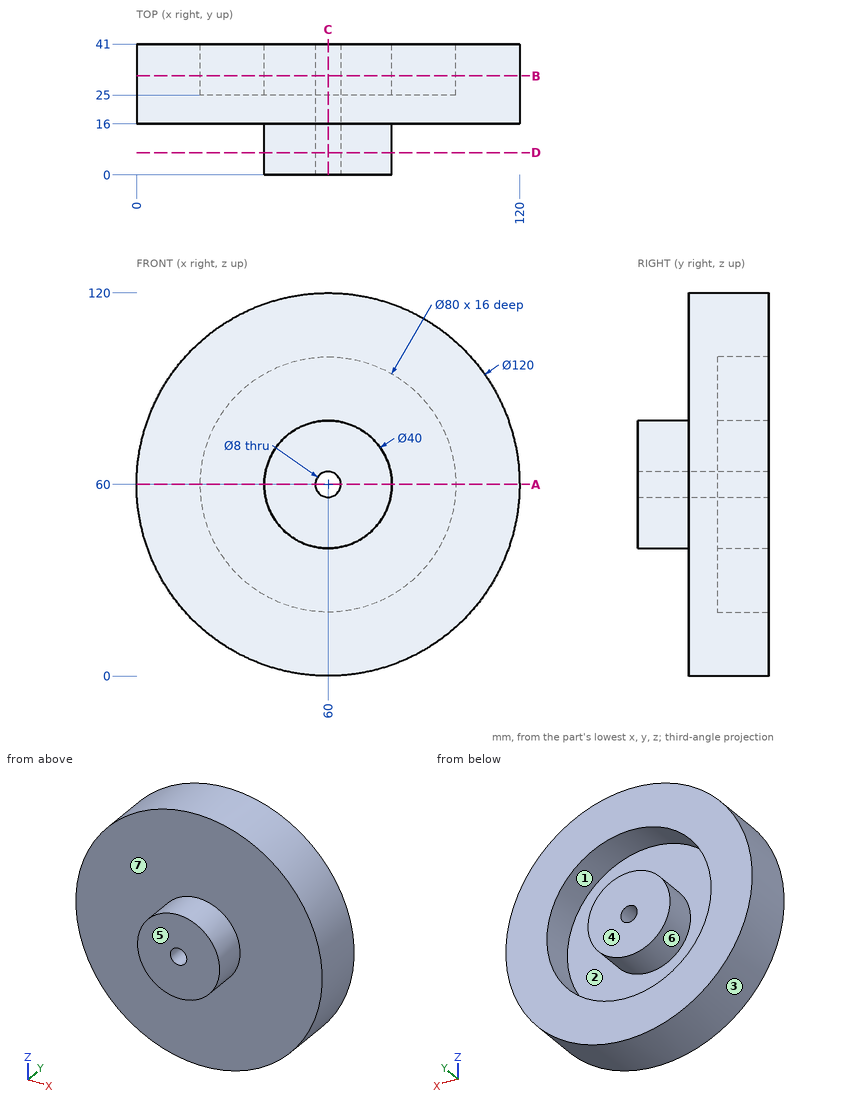
The drawing under review shows one solid part. Ordinate dimensions are in mm from its lowest x, y, z. A direction names the side the tool comes from. Round coordinates to 2 decimals unless told otherwise and drop trailing zeros. Write each loop counter-clockwise with the first axis right and the second up, starting at its lowest first coordinate (ties: lowest second). Pieces come first, ordered by that corner, then holes.
(1) We need section A-A on z = 60. Give the boundary of the cut face in (x, y).
(2) Machinability: for the marked faces 5, 6 and 7, which of the approach directions +Z, -Z, +X, -X, +Y, -Y give a long, thin tool a straight path to every point of the face, cutting with its end or side? Answer none if there is none.
(3) Wall thickness on L1, parallel to X at y = 30.5, z = 60; L2, parallel to X at y = 12, z = 60; L3, parallel to Y at x = 8.5, z = 67.5: over which ranges is each line inside the solid? List them lowest first.
(4) Mouldability with a two-part tool opening along X and no side actions: class the marked faces 1, 2, 3 and 4 as +X half, -X half, draft (parallel to the pull), parting line (faces both ways), or undercut.
(5) We need section D-D on y = 7. Give the boundary of the cut face in (x, z), and give its area (3 significant figures).
(6) Insertion check: pin 1 (1.5 mm diameter, centred on x = 100, y = 22, fed in from -Z); pin 2 (12 mm diameter, centred on x = 12, z = 73, fed in from -Y); pin 3 (6 mm diameter, centred on x = 50.5, y = 9, fed in from -Z). Each pin has a flat end and moves straight along its axis. Give the tip position at first contact, or say it passes through.
(7) We need section C-C on x = 60. Give the boundary of the cut face in (y, z).
(8) We need section B-B on y = 31. Give the boundary of the cut face in (x, z), and give its area (3 significant figures).
Findings below:
1. outline: (0, 16) - (40, 16) - (40, 0) - (56, 0) - (56, 41) - (40, 41) - (40, 25) - (20, 25) - (20, 41) - (0, 41) - close; (64, 0) - (80, 0) - (80, 16) - (120, 16) - (120, 41) - (100, 41) - (100, 25) - (80, 25) - (80, 41) - (64, 41) - close
2. face 5: +Z, -Z, +X, -X, -Y
2. face 6: +Y
2. face 7: -Y
3. L1: x = 0 to 20, 40 to 56, 64 to 80, 100 to 120
3. L2: x = 40 to 56, 64 to 80
3. L3: y = 16 to 41
4. face 1: undercut
4. face 2: undercut
4. face 3: parting line
4. face 4: draft
5. outline: circle Ø40 at (60, 60); hole circle Ø8 at (60, 60)
5. area: 1,210 mm2
6. pin 1: stops at z = 14.62
6. pin 2: stops at y = 16
6. pin 3: stops at z = 41.09
7. outline: (0, 40) - (16, 40) - (16, 0) - (41, 0) - (41, 20) - (25, 20) - (25, 40) - (41, 40) - (41, 56) - (0, 56) - close; (0, 64) - (41, 64) - (41, 80) - (25, 80) - (25, 100) - (41, 100) - (41, 120) - (16, 120) - (16, 80) - (0, 80) - close
8. outline: circle Ø120 at (60, 60); circle Ø40 at (60, 60); hole circle Ø80 at (60, 60); hole circle Ø8 at (60, 60)
8. area: 7,490 mm2
